Geometry: final body of the model. Coordinates: model frame, mm. Give positions to 0.01 mm unless a question says otherwise; leave off trailing zeros. Write each loop counter-clockwise with the first axis right and the second up, starting at its lowest first coordinate (ties: lowest second). Pieces come first, ordered by that corner, then holes. Notation, with made-up numbers: (89.5, 15) -> (126.5, 15) arc R26 cw to (126.5, 41) -> close; hole circle Ø8 at (46.5, -5). An arc over 180 degrees is marked (long way). Answer as a JSON object with one key per item and string values. Group by question number.
(1) Section query B-B on x = 10.75. Output: boundary loops of the cut face in (y, z), plus the area to 3 significant figures.
(2) Section query A-A on z = 4.4. Output: boundary loops of the cut face in (x, y), plus the area to 3 significant figures.
(3) Section query C-C on x = 24. Output: boundary loops of the cut face in (y, z), plus the area to 3 significant figures.
(4) Section query D-D on y = -7. Output: boundary loops of the cut face in (x, z), plus the area to 3 significant figures.
(5) Contact query for flat-ended pins moving along their axis: pin 1 Ø2 at (x, z) = (19.5, 4.5) entering from -Y; pin 2 Ø2 at (y, z) = (-13, 4.5) entering from +X; pin 3 Ø1.8 at (y, z) = (-23.7, 3.3) entering from +X; pin 4 Ø0.5 at (x, z) = (26.5, 1) entering from +Y. Output: stop coordinate, or through.
(6) Material intervals for probe 1 along Y at (x, z) = (14.75, 3.3); probe 2 along X at (y, z) = (0.25, 4.05); probe 3 along Y at (x, z) = (1.25, 0.7), sorted ascending.
from build123d import *

# Parameters (mm, degrees)
SKETCH_1_W          = 28
SKETCH_1_H          = 25.2
EXTRUDE_1_DEPTH     = 1.8
SKETCH_2_W          = 11.8
SKETCH_2_H          = 3
EXTRUDE_2_DEPTH     = 3
FILLET_1_R          = 1.4
SKETCH_3_R          = 0.55
CUT_EXTRUDE_1_DEPTH = 20.9
SKETCH_4_W          = 6.4
SKETCH_4_H          = 1.8
EXTRUDE_3_DEPTH     = 1.5
SKETCH_5_W          = 6.4
SKETCH_5_H          = 1.5
EXTRUDE_4_DEPTH     = 3.6
SKETCH_7_R          = 1
EXTRUDE_5_DEPTH     = 6.4
SKETCH_8_R          = 1
EXTRUDE_6_DEPTH     = 6.4


with BuildPart() as part:
    # 草图1 → 凸台-拉伸1 (new body)
    with BuildSketch(Plane.XY):
        with Locations((14, -12.6)):
            Rectangle(SKETCH_1_W, SKETCH_1_H)
    extrude(amount=EXTRUDE_1_DEPTH)

    # 草图2 → 凸台-拉伸2 (add)
    with BuildSketch(Plane.XY.offset(1.8)):
        with Locations((14, -23.7)):
            Rectangle(SKETCH_2_W, SKETCH_2_H)
    extrude(amount=EXTRUDE_2_DEPTH)

    # 圆角1
    fillet_1_edges = [part.edges().sort_by_distance(p)[0] for p in [
        (14, -25.2, 4.8),
        (14, -22.2, 4.8),
    ]]
    fillet(fillet_1_edges, radius=FILLET_1_R)

    # 草图3 → 切除-拉伸1 (cut, through all)
    with BuildSketch(Plane(origin=(19.9, 0, 0), x_dir=(0, 0, -1), z_dir=(1, 0, 0))):
        with Locations((-3.3, -23.7)):
            Circle(SKETCH_3_R)
    extrude(amount=-CUT_EXTRUDE_1_DEPTH, mode=Mode.SUBTRACT)

    # 草图4 → 凸台-拉伸3 (add)
    with BuildSketch(Plane(origin=(0, 0, 0), x_dir=(1, 0, 0), z_dir=(0, 1, 0))):
        with Locations((5.5, -0.9)):
            Rectangle(SKETCH_4_W, SKETCH_4_H)
        with Locations((22.5, -0.9)):
            Rectangle(SKETCH_4_W, SKETCH_4_H)
    extrude(amount=EXTRUDE_3_DEPTH)

    # 草图5 → 凸台-拉伸4 (add)
    with BuildSketch(Plane.XY.offset(1.8)):
        with Locations((5.5, 0.75)):
            Rectangle(SKETCH_5_W, SKETCH_5_H)
        with Locations((22.5, 0.75)):
            Rectangle(SKETCH_5_W, SKETCH_5_H)
    extrude(amount=EXTRUDE_4_DEPTH)

    # 草图7 → 凸台-拉伸5 (add)
    with BuildSketch(Plane(origin=(25.7, 0, 0), x_dir=(0, 0, -1), z_dir=(1, 0, 0))):
        with Locations((-4.4, 0)):
            Circle(SKETCH_7_R)
    extrude(amount=-EXTRUDE_5_DEPTH)

    # 草图8 → 凸台-拉伸6 (add)
    with BuildSketch(Plane.ZY.offset(-2.3)):
        with Locations((4.4, 0)):
            Circle(SKETCH_8_R)
    extrude(amount=-EXTRUDE_6_DEPTH)


solid = part.part
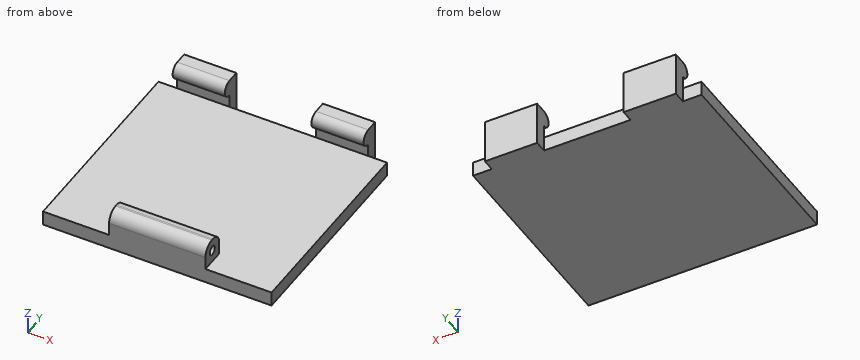
Answer list:
{
 "1": {"outline": "(-25.2, 0) -> (0, 0) -> (0, 1.8) -> (-22.2, 1.8) -> (-22.2, 3.4) arc R1.4 ccw to (-23.6, 4.8) -> (-23.8, 4.8) arc R1.4 ccw to (-25.2, 3.4) -> close; hole circle Ø1.1 at (-23.7, 3.3)", "area": "52.6 mm2"},
 "2": {"outline": "(2.3, -1) -> (8.7, -1) -> (8.7, 1.5) -> (2.3, 1.5) -> close; (8.1, -24.78) -> (19.9, -24.78) -> (19.9, -22.62) -> (8.1, -22.62) -> close; (19.3, -1) -> (25.7, -1) -> (25.7, 1.5) -> (19.3, 1.5) -> close", "area": "57.5 mm2"},
 "3": {"outline": "(-25.2, 0) -> (1.5, 0) -> (1.5, 5.4) -> (0, 5.4) arc R1 ccw to (0, 3.4) -> (0, 1.8) -> (-25.2, 1.8) -> close", "area": "55.0 mm2"},
 "4": {"outline": "(0, 0) -> (28, 0) -> (28, 1.8) -> (0, 1.8) -> close", "area": "50.4 mm2"},
 "5": {"pin 1": "y = -25.2", "pin 2": "through", "pin 3": "x = 19.9", "pin 4": "y = 0"},
 "6": {"probe 1": "-25.2 to -24.25, -23.15 to -22.2", "probe 2": "2.3 to 8.7, 19.3 to 25.7", "probe 3": "-25.2 to 0"}
}
